Here's how the part is built. I have some questions about the finished solid (model axes, mm). Face numbers are marked on the shaded views. A direction names the side the tool comes from. Round coordinates to 2 decimals unless told otherwise and drop trailing zeros. Order: outer loops, then holes, each group sorted by start corner. A loop starts at its lowest first (then second) coordinate and runs counter-clockwise, first axis right, second up. Notation, with made-up numbers: (2, 18) -> (9, 18) arc R22 cw to (9, 24) -> close; hole circle Ø11 at (-25.5, -5.5). An arc over 180 degrees is marked (long way). Answer in a Markdown table with one row per item.
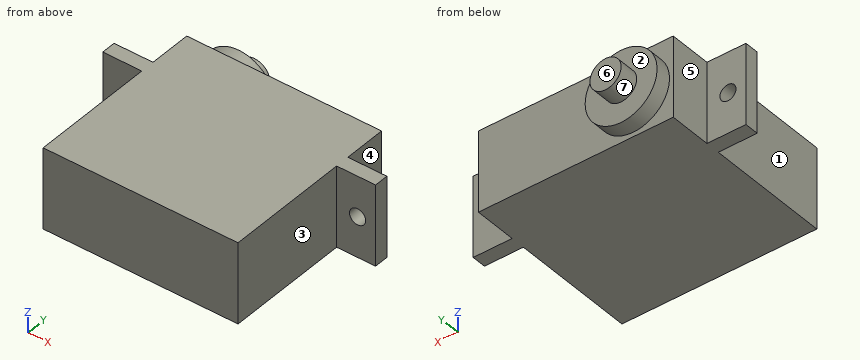
```python
from build123d import *

# Parameters (mm, degrees)
BOSS_EXTRUDE1_DEPTH = 4.98
SKETCH2_R           = 0.99
CUT_EXTRUDE1_DEPTH  = 18.1
SKETCH3_R           = 4.42938454
BOSS_EXTRUDE2_DEPTH = 1.93
SKETCH4_R           = 1.916429151
BOSS_EXTRUDE3_DEPTH = 2.43


with BuildPart() as part:
    # Sketch1 → Boss-Extrude1 (new body, symmetric)
    with BuildSketch(Plane.XY):
        Polygon((19.1, 1.75), (23.9, 1.75), (23.9, 0), (19.1, 0), (19.1, -15.35), (-4.9, -15.35), (-4.9, 0), (-9.7, 0), (-9.7, 1.75), (-4.9, 1.75), (-4.9, 7), (19.1, 7), align=None)
    extrude(amount=BOSS_EXTRUDE1_DEPTH, both=True)

    # Sketch2 → Cut-Extrude1 (cut, through all)
    with BuildSketch(Plane(origin=(0, 1.75, 0), x_dir=(1, 0, 0), z_dir=(0, 1, 0))):
        with Locations((-7.48, 0)):
            Circle(SKETCH2_R)
        with Locations((21.68, 0)):
            Circle(SKETCH2_R)
    extrude(amount=-CUT_EXTRUDE1_DEPTH, mode=Mode.SUBTRACT)

    # Sketch3 → Boss-Extrude2 (add)
    with BuildSketch(Plane(origin=(0, 7, 0), x_dir=(1, 0, 0), z_dir=(0, 1, 0))):
        Circle(SKETCH3_R)
    extrude(amount=BOSS_EXTRUDE2_DEPTH)

    # Sketch4 → Boss-Extrude3 (add)
    with BuildSketch(Plane(origin=(0, 8.93, 0), x_dir=(1, 0, 0), z_dir=(0, 1, 0))):
        Circle(SKETCH4_R)
    extrude(amount=BOSS_EXTRUDE3_DEPTH)


solid = part.part
```
1. Suppose I cut it at A-A on x = -7.48. Write out the boundary of the cut face in (y, z), then the cut area to 3 significant figures.
Numbers:
| item | result |
|---|---|
| outline | (0, -4.98) -> (1.75, -4.98) -> (1.75, -0.99) -> (0, -0.99) -> close; (0, 0.99) -> (1.75, 0.99) -> (1.75, 4.98) -> (0, 4.98) -> close |
| area | 14.0 mm2 |
2. Please list where these lines run through material, in increasing order: line 1 along X through (y, z) = (1.1, 0); line 2 along Z through (x, y) = (-7.48, 1.25); line 3 along Y through (x, z) = (21, 1.5).
Numbers:
| item | result |
|---|---|
| line 1 | x = -9.7 to -8.47, -6.49 to 20.69, 22.67 to 23.9 |
| line 2 | z = -4.98 to -0.99, 0.99 to 4.98 |
| line 3 | y = 0 to 1.75 |
3. For pin 1 Ø2.5 at (x, z) = (-7.48, 0) entering from +Y; pin 2 Ø5.5 at (x, z) = (-6.5, 1.5) entering from +Y; pin 3 Ø1.5 at (y, z) = (7.5, -1.5) entering from +X; pin 4 Ø4 at (x, z) = (-6.5, 1) entering from -Y, each with a flat end and sliding along its axis, tell me the tip position at first contact or that it passes through.
Numbers:
| item | result |
|---|---|
| pin 1 | stops at y = 1.75 |
| pin 2 | stops at y = 8.93 |
| pin 3 | stops at x = 19.1 |
| pin 4 | stops at y = -15.35 |
4. We'd pull the mould along X, two halves only. Please class the marked faces 4, 5, 6 and 7: released by +X, released by -X, zero draft, split by the parting line, or undercut.
Numbers:
| item | result |
|---|---|
| face 4 | released by +X |
| face 5 | released by -X |
| face 6 | zero draft |
| face 7 | split by the parting line |
5. Suppose I cut it at C-C on x = 0. Write out the boundary of the cut face in (y, z), then the cut area to 3 significant figures.
Numbers:
| item | result |
|---|---|
| outline | (-15.35, -4.98) -> (7, -4.98) -> (7, -4.43) -> (8.93, -4.43) -> (8.93, -1.92) -> (11.36, -1.92) -> (11.36, 1.92) -> (8.93, 1.92) -> (8.93, 4.43) -> (7, 4.43) -> (7, 4.98) -> (-15.35, 4.98) -> close |
| area | 249 mm2 |
6. For the marked faces 1, 2 and 3, which set-ups out of +Z, -Z, +X, -X, +Y, -Y let a thin tool reach every point of the face, with its end or its side?
Numbers:
| item | result |
|---|---|
| face 1 | +Z, -Z, -X, -Y |
| face 2 | +Y |
| face 3 | +Z, -Z, +X, -Y |
7. Suppose I cut it at B-B on z = 0. Write out the boundary of the cut face in (x, y).
Numbers:
| item | result |
|---|---|
| outline | (-9.7, 0) -> (-8.47, 0) -> (-8.47, 1.75) -> (-9.7, 1.75) -> close; (-6.49, 0) -> (-4.9, 0) -> (-4.9, -15.35) -> (19.1, -15.35) -> (19.1, 0) -> (20.69, 0) -> (20.69, 1.75) -> (19.1, 1.75) -> (19.1, 7) -> (4.43, 7) -> (4.43, 8.93) -> (1.92, 8.93) -> (1.92, 11.36) -> (-1.92, 11.36) -> (-1.92, 8.93) -> (-4.43, 8.93) -> (-4.43, 7) -> (-4.9, 7) -> (-4.9, 1.75) -> (-6.49, 1.75) -> close; (22.67, 0) -> (23.9, 0) -> (23.9, 1.75) -> (22.67, 1.75) -> close |
8. Suppose I cut it at D-D on z = -3.5. Write out the boundary of the cut face in (x, y).
Numbers:
| item | result |
|---|---|
| outline | (-9.7, 0) -> (-4.9, 0) -> (-4.9, -15.35) -> (19.1, -15.35) -> (19.1, 0) -> (23.9, 0) -> (23.9, 1.75) -> (19.1, 1.75) -> (19.1, 7) -> (2.71, 7) -> (2.71, 8.93) -> (-2.71, 8.93) -> (-2.71, 7) -> (-4.9, 7) -> (-4.9, 1.75) -> (-9.7, 1.75) -> close |
